Can you work these out from the drawing? Everything is in mm from the part's minimum corner. Round coordinates to 2 decimals unless told otherwise and drop trailing zeros. Write each loop counter-clockwise with the first axis right and the second up, starting at its lowest first coordinate (ties: lowest second). Pieces come first, ordered by that corner, then holes.
Q1. If we section it at C-C (y = 485.5): Please give me the cut outline in (x, z), plus the area to 3 significant figures.
Q2. If we section it at B-B (x = 700): Please give me the cut outline in (y, z), plus the area to 3 significant figures.
Q3. We'd pull the mould along X, two halves only. Please class the marked faces 1, 2 and 3: +X half, -X half, draft (parallel to the pull), parting line (faces both ways), or undercut.
Q4. I'm going to push a flat-ended pin straight in: pin 1 Ø1.5 at (y, z) = (83.5, 892) entering from -X. Where does the tip first touch, or does it pass through?
Q5. Please list where these lines run through material, in increasing order: line 1 along X through (y, z) = (528.5, 700); line 2 along Y through (x, z) = (481.5, 615).
Q6. If we section it at A-A (z = 700): Please give me the cut outline in (x, y).
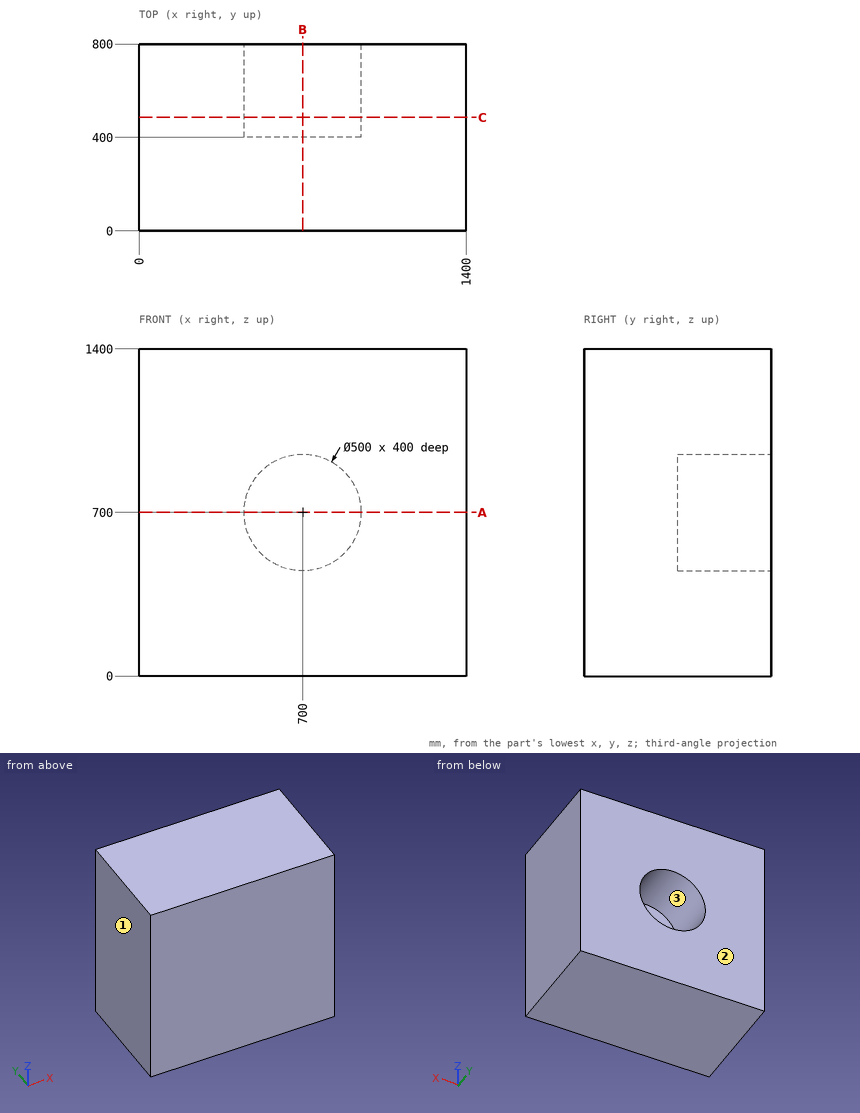
A:
1. outline: (0, 0) - (1400, 0) - (1400, 1400) - (0, 1400) - close; hole circle Ø500 at (700, 700)
1. area: 1,760,000 mm2
2. outline: (0, 0) - (800, 0) - (800, 450) - (400, 450) - (400, 950) - (800, 950) - (800, 1400) - (0, 1400) - close
2. area: 920,000 mm2
3. face 1: -X half
3. face 2: draft
3. face 3: undercut
4. pin 1: stops at x = 0
5. line 1: x = 0 to 450, 950 to 1400
5. line 2: y = 0 to 400
6. outline: (0, 0) - (1400, 0) - (1400, 800) - (950, 800) - (950, 400) - (450, 400) - (450, 800) - (0, 800) - close
